from build123d import *

# Parameters (mm, degrees)
SM_BASE_FLANGE_1_DEPTH = 50


# Sheet-metal steps are written as plain solids
with BuildPart() as part:
    # Sketch 1 → Базовая кромка1 (new body)
    with BuildSketch(Plane.XY):
        with BuildLine():
            Line((0, 0), (0, 16))
            ThreePointArc((0, 16), (1.171572875, 18.828427125), (4, 20))
            Line((4, 20), (44, 20))
            ThreePointArc((44, 20), (46.828427125, 18.828427125), (48, 16))
            Line((48, 16), (48, 0))
            Line((48, 0), (46, 0))
            Line((46, 0), (46, 16))
            ThreePointArc((46, 16), (45.414213562, 17.414213562), (44, 18))
            Line((44, 18), (4, 18))
            ThreePointArc((4, 18), (2.585786438, 17.414213562), (2, 16))
            Line((2, 16), (2, 0))
            Line((2, 0), (0, 0))
        make_face()
    extrude(amount=-SM_BASE_FLANGE_1_DEPTH)


solid = part.part
Check sheet for the modelled part. Datum: model origin and axes. Units: mm. A direction names the side the tool comes from. Give positions to 0.01 mm unless a question says otherwise; leave off trailing zeros. Write each loop counter-clockwise with the first axis right and the second up, starting at its lowest first coordinate (ties: lowest second). Pieces come first, ordered by that corner, then holes. Notation, with made-up numbers: (56, -36.5) -> (108, -36.5) arc R7 cw to (108, -27.5) -> close; hole circle Ø11 at (-21, 20.25). An arc over 180 degrees is marked (long way). One line per item, written item: value. Start each with the question number.
Item 1: Section check C-C on x = 33.5. Record the cut outline in (y, z).
Item 2: Draft check along X on faces 3 (the flat face through (1, 0, -25)), 4 (the cylindrical face through (1.141, 18.797, -24.65)), 5 (the flat face through (46, 8, -25)), 6 (the cylindrical face through (45.43, 17.4, -24.65)). Enter one of: +X half, -X half, draft (parallel to the pull), parting line (faces both ways), or undercut.
Item 3: Tool access check on faces 1 (the cylindrical face through (46.797, 18.859, -24.65)), 2 (the flat face through (2, 8, -25)). Record the directions out of +Z, -Z, +X, -X, +Y, -Y that give a thin tool (end or side, any length) a straight path to the whole face; none if there is none.
Item 4: Section check B-B on z = -20.5. Record the cut outline in (x, y), then the cut area to 3 significant figures.
Item 5: Gauge pin test, flat end, axial feed: pin 1 (1.5 mm diameter, centred on x = 24.5, z = -25.5, fed in from -Y). Record the tip position at first contact, or that the pin passes through.
Item 6: Section check A-A on y = 8.75. Record the cut outline in (x, z).
Item 7: Material ranges on probe 1 along X at (y, z) = (9.5, -3); probe 2 along Y at (x, z) = (27.5, -31); probe 3 along X at (y, z) = (18.75, -29), recorded low to high. Write a range as from..to.
Item 8: Section check D-D on x = 3. Record the cut outline in (y, z).
Results list:
1. outline: (18, -50) -> (20, -50) -> (20, 0) -> (18, 0) -> close
2. face 3: draft
2. face 4: -X half
2. face 5: undercut
2. face 6: undercut
3. face 1: +Z, -Z, +X, +Y
3. face 2: +Z, -Z, -Y
4. outline: (0, 0) -> (2, 0) -> (2, 16) arc R2 cw to (4, 18) -> (44, 18) arc R2 cw to (46, 16) -> (46, 0) -> (48, 0) -> (48, 16) arc R4 ccw to (44, 20) -> (4, 20) arc R4 ccw to (0, 16) -> close
4. area: 163 mm²
5. pin 1: y = 18
6. outline: (0, -50) -> (2, -50) -> (2, 0) -> (0, 0) -> close; (46, -50) -> (48, -50) -> (48, 0) -> (46, 0) -> close
7. probe 1: 0..2, 46..48
7. probe 2: 18..20
7. probe 3: 1.1..46.9
8. outline: (17.73, -50) -> (19.87, -50) -> (19.87, 0) -> (17.73, 0) -> close
